Design review of the part built by this model. Coordinates are the model's own, in mm. A direction names the side the tool comes from. Give positions to 0.01 mm unless a question says otherwise; leave off trailing zeros. Loops run counter-clockwise (first coordinate to the right, second up) from the corner with the lowest first, then second, coordinate; pieces in that order, holes last. Notation, with made-up numbers: (37, 34.25) -> (66, 34.25) arc R29 cw to (66, 54.25) -> close; hole circle Ø2 at (3, 88.5). An arc over 180 degrees is marked (long way). Use a Markdown table: item, result. Add a question column.
1. Add section C-C (x = 35). Count the separate pieces of the cut face and the enclosed holes in it, and give its area (3 significant figures).
2. Add section B-B (x = -35). State the section outline as (y, z) points, and give its area (3 significant figures).
3. Draft analysis for pull direction Z (two halves, no side actions). For faces 5 (the cylindrical face through (129.529, 134.897, 79.997)), 6 (the cylindrical face through (129.529, 142.036, 65.976)), 7 (the cylindrical face through (129.529, 134.302, -79.997)), state which applies: pulls with the +Z half, pulls with the -Z half, needs draft (parallel to the pull), parting line crosses it, or undercut.
4. For pin 1 Ø13.5 at (y, z) = (134.6, -65) entering from +X; pin 2 Ø16 at (x, z) = (0, -35) entering from -Y; pin 3 Ø11.5 at (x, z) = (35, 0) entering from +Y; pin 4 Ø24.5 at (y, z) = (143, 44) entering from -X, all flat-tipped, find the tip position at first contact; note any pin that passes through.
5. Add section A-A (z = 35). State the section outline as (x, y) points.
6. For faces 1 (the flat face through (134.599, 118, 19)), 2 (the cylindrical face through (-8.618, 4.93, 20.784)), 3 (the flat face through (129.529, 114.907, 36.021)), 4 (the flat face through (129.529, 114.768, -35.133)), list the 3-axis set-ups (+Z, -Z, +X, -X, +Y, -Y) from which the entire face can be reached by the end or side of a thin tool; tool diameter is ignored.
7. To check wall thickness, follow line 1 (X direction, y = 2.5, z = 0); line 2 (Z direction, x = 57, y = 124); line 3 (Y direction, x = 6, z = 32.5). State the ranges of each line that lie inside material, in increasing order.
```python
from build123d import *

# Parameters (mm, degrees)
SKETCH1_R           = 45
SKETCH1_R_2         = 5
SKETCH1_R_3         = 22.5
BOSS_EXTRUDE1_DEPTH = 10
SKETCH3_R           = 25
SKETCH3_R_2         = 22.5
SKETCH4_R           = 7.5
SKETCH4_R_2         = 25
SKETCH4_R_3         = 22.5
BOSS_EXTRUDE6_DEPTH = 10


with BuildPart() as part:
    # Sketch1 → Boss-Extrude1 (new body)
    with BuildSketch(Plane(origin=(0, 0, 0), x_dir=(1, 0, 0), z_dir=(0, 1, 0))):
        with Locations(Location((0, 0, 0), (0, 0, 270))):
            Circle(SKETCH1_R)
        with Locations(Location((0, 35, 0), (0, 0, 270))):
            Circle(SKETCH1_R_2, mode=Mode.SUBTRACT)
        with Locations(Location((35, 0, 0), (0, 0, 270))):
            Circle(SKETCH1_R_2, mode=Mode.SUBTRACT)
        with Locations(Location((0, -35, 0), (0, 0, 270))):
            Circle(SKETCH1_R_2, mode=Mode.SUBTRACT)
        with Locations(Location((-35, 0, 0), (0, 0, 270))):
            Circle(SKETCH1_R_2, mode=Mode.SUBTRACT)
        with Locations(Location((0, 0, 0), (0, 0, 270))):
            Circle(SKETCH1_R_3, mode=Mode.SUBTRACT)
    extrude(amount=BOSS_EXTRUDE1_DEPTH)

    # Sweep1: sweep along a path in Sketch2
    with BuildLine(Plane.XY) as sweep1_path:
        ThreePointArc((124.599357944, 135), (36.211010295, 98.388347648), (-0.400642056, 10))
    # Sketch3 → Sweep1 (sweep)
    with BuildSketch(Plane(origin=(0, 10, 0), x_dir=(1, 0, 0), z_dir=(0, 1, 0))):
        Circle(SKETCH3_R)
        Circle(SKETCH3_R_2, mode=Mode.SUBTRACT)
    sweep(path=sweep1_path.line)

    # Sketch4 → Boss-Extrude6 (add)
    # profile 1 of 3: a face of its own
    with BuildSketch(Plane(origin=(124.599357944, 0, 0), x_dir=(0, 0, -1), z_dir=(1, 0, 0))):
        with BuildLine():
            ThreePointArc((-3.846153846, 109.8969876), (-25, 134.599357944), (-3.846153846, 159.301728287))
            Line((-3.846153846, 159.301728287), (-67.307692308, 149.42078015))
            ThreePointArc((-67.307692308, 149.42078015), (-80, 134.599357944), (-67.307692308, 119.777935738))
            Line((-67.307692308, 119.777935738), (-3.846153846, 109.8969876))
        make_face()
        with Locations((-65, 134.599357944)):
            Circle(SKETCH4_R, mode=Mode.SUBTRACT)
    # profile 2 of 3: a face of its own
    with BuildSketch(Plane(origin=(124.599357944, 0, 0), x_dir=(0, 0, -1), z_dir=(1, 0, 0))):
        with BuildLine():
            Line((67.307692308, 149.42078015), (3.846153846, 159.301728287))
            ThreePointArc((3.846153846, 159.301728287), (18.988863133, 150.860448833), (25, 134.599357944))
            ThreePointArc((25, 134.599357944), (18.988863133, 118.338267054), (3.846153846, 109.8969876))
            Line((3.846153846, 109.8969876), (67.307692308, 119.777935738))
            ThreePointArc((67.307692308, 119.777935738), (80, 134.599357944), (67.307692308, 149.42078015))
        make_face()
        with Locations((65, 134.599357944)):
            Circle(SKETCH4_R, mode=Mode.SUBTRACT)
    # profile 3 of 3: a face of its own
    with BuildSketch(Plane(origin=(124.599357944, 0, 0), x_dir=(0, 0, -1), z_dir=(1, 0, 0))):
        with Locations((0, 134.599357944)):
            Circle(SKETCH4_R_2)
        with Locations(Location((0, 134.599357944, 0), (0, 0, 90))):
            Circle(SKETCH4_R_3, mode=Mode.SUBTRACT)
    extrude(amount=BOSS_EXTRUDE6_DEPTH)


solid = part.part
```
Taken from the geometry:
| question | item | result |
|---|---|---|
| 1 | separate pieces | 3 |
| 1 | enclosed holes | 1 |
| 1 | area | 1,050 mm^2 |
| 2 | outline | (0, -28.28) -> (10, -28.28) -> (10, -5) -> (0, -5) -> close; (0, 5) -> (10, 5) -> (10, 28.28) -> (0, 28.28) -> close |
| 2 | area | 466 mm^2 |
| 3 | face 5 | pulls with the +Z half |
| 3 | face 6 | undercut |
| 3 | face 7 | pulls with the -Z half |
| 4 | pin 1 | passes through |
| 4 | pin 2 | stops at y = 0 |
| 4 | pin 3 | stops at y = 133.89 |
| 4 | pin 4 | stops at x = 124.6 |
| 5 | outline | (-28.28, 0) -> (-5, 0) -> (-5, 10) -> (-28.28, 10) -> close; (5, 0) -> (28.28, 0) -> (28.28, 10) -> (5, 10) -> close; (124.6, 114.75) -> (134.6, 114.75) -> (134.6, 154.45) -> (124.6, 154.45) -> close |
| 6 | face 1 | +Z, -Z, +X, +Y, -Y |
| 6 | face 2 | -Y |
| 6 | face 3 | +Z, +X, -Y |
| 6 | face 4 | -Z, +X, -Y |
| 7 | line 1 | x = -45 to -40, -30 to -22.5, 22.5 to 30, 40 to 45 |
| 7 | line 2 | z = -23.71 to -21.05, 21.05 to 23.71 |
| 7 | line 3 | y = 0 to 10 |
